Read the model definition and answer for the solid it produces. Units are mm, in the model's axes. A direction names the side the tool comes from. Give positions to 0.01 mm unless a question says otherwise; leave off trailing zeros. Write each loop counter-clockwise with the first axis right and the second up, starting at its lowest first coordinate (ties: lowest second). Pieces come first, ordered by that corner, then holes.
```python
from build123d import *

# Parameters (mm, degrees)
F1_DEPTH      = 3.5
F0_W          = 1.25
F0_H          = 11.5
F2_W          = 21
F2_H          = 11.5
F3_DEPTH      = 2
F4_W          = 27
F4_H          = 14.5
F4_W_2        = 21
F4_H_2        = 5.5
F5_DEPTH      = 11.5
F5_DEPTH_BACK = 4
F6_R          = 1.75
F7_DEPTH      = 25
F9_DEPTH      = 4
F10_R         = 3
F11_DEPTH     = 3
F12_SIZE      = 0.9999
F13_R         = 1.75
F14_DEPTH     = 5


# Not quite as in the source:
# - a fillet or chamfer is up to 0.001 mm smaller than in the source, because OpenCascade refuses the exact size


with BuildPart() as f1:
    # F0 (on Top) → F1 (new body)
    with BuildSketch(Plane.XY):
        Polygon((1.25, 0), (0, 0), (-1.25, 0), (-1.25, -11.5), (0, -11.5), (1.25, -11.5), align=None)
    extrude(amount=F1_DEPTH)



with BuildPart() as f1b:
    # F0 (on Top) → F1, piece 2 (new body)
    with BuildSketch(Plane.XY):
        with Locations((-9.875, -5.75)):
            Rectangle(F0_W, F0_H)
    extrude(amount=F1_DEPTH)


with BuildPart() as f1c:
    # F0 (on Top) → F1, piece 3 (new body)
    with BuildSketch(Plane.XY):
        with Locations((9.875, -5.75)):
            Rectangle(F0_W, F0_H)
    extrude(amount=F1_DEPTH)


with BuildPart() as f1_1:
    add(f1.part)

    add(f1b.part)  # F3 merges F1b

    add(f1c.part)  # F3 merges F1c
    # F2 (on Top) → F3 (join)
    with BuildSketch(Plane.XY):
        with Locations((0, -5.75)):
            Rectangle(F2_W, F2_H)
    extrude(amount=-F3_DEPTH)

    # F4 (on Front) → F5 (join, two sides)
    with BuildSketch(Plane.XZ) as f5_sk:
        with Locations((0, 2.25)):
            Rectangle(F4_W, F4_H)
        with Locations((0, 0.75)):
            Rectangle(F4_W_2, F4_H_2, mode=Mode.SUBTRACT)
    extrude(amount=F5_DEPTH)
    extrude(f5_sk.sketch, amount=-F5_DEPTH_BACK)

    # F6 (on face) → F7 (cut)
    with BuildSketch(Plane.XY):
        with Locations((5.25, -7.5)):
            Circle(F6_R)
        with Locations((-5.25, -7.5)):
            Circle(F6_R)
    extrude(amount=F7_DEPTH, mode=Mode.SUBTRACT)

    # F8 (on face) → F9 (cut)
    with BuildSketch(Plane(origin=(0, 0, 3.5), x_dir=(1, 0, 0), z_dir=(0, 0, -1))):
        Polygon((2.25, 5.7679491924), (5.25, 4.0358983849), (8.25, 5.7679491924), (8.25, 9.2320508076), (5.25, 10.9641016151), (2.25, 9.2320508076), align=None)
        Polygon((2.25, 21.0246167397), (2.25, 9.2320508076), (5.25, 10.9641016151), (8.25, 9.2320508076), (8.25, 21.0246167397), align=None)
        Polygon((-2.25, 21.0246167397), (-8.25, 21.0246167397), (-8.25, 9.2320508076), (-8.25, 5.7679491924), (-5.25, 4.0358983849), (-2.25, 5.7679491924), (-2.25, 9.2320508076), align=None)
    extrude(amount=-F9_DEPTH, mode=Mode.SUBTRACT)

    # F10 (on face) → F11 (cut)
    with BuildSketch(Plane.XZ.offset(11.5)):
        with Locations((5.25, 1.75)):
            Circle(F10_R)
        with Locations((-5.25, 1.75)):
            Circle(F10_R)
    extrude(amount=-F11_DEPTH, mode=Mode.SUBTRACT)

    # F12 (size 1 in the source; OpenCascade refuses exactly that, so slightly less here)
    f12_edges = [f1_1.edges().sort_by_distance(p)[0] for p in [
        (-1.25, -11.5, 1.75),
        (-9.25, -11.5, 1.75),
        (-2.031651, -11.5, 0),
        (-8.468349, -11.5, 0),
        (2.031651, -11.5, 0),
        (1.25, -11.5, 1.75),
        (5.25, -11.5, -1.25),
        (8.468349, -11.5, 0),
        (9.25, -11.5, 1.75),
        (-5.25, -11.5, -1.25),
        (-8.25, -11.5, 5.5),
        (-5.25, -11.5, 7.5),
        (-2.25, -11.5, 5.5),
        (2.25, -11.5, 5.5),
        (5.25, -11.5, 7.5),
        (8.25, -11.5, 5.5),
    ]]
    chamfer(f12_edges, length=F12_SIZE)

    # F13 (on face) → F14 (join)
    with BuildSketch(Plane(origin=(0, 0, -5), x_dir=(1, 0, 0), z_dir=(0, 0, -1))):
        with BuildLine():
            Line((13.5, -4), (17.5, -4))
            ThreePointArc((17.5, -4), (25.25, 3.75), (17.5, 11.5))
            Line((17.5, 11.5), (13.5, 11.5))
            Line((13.5, 11.5000000001), (13.5, -4))
        make_face()
        with Locations((17.5, 3.75)):
            Circle(F13_R, mode=Mode.SUBTRACT)
        with BuildLine():
            ThreePointArc((-17.5, 11.5), (-25.25, 3.75), (-17.5, -4))
            Line((-17.5, -4), (-13.5, -4))
            Line((-13.5, -4), (-13.5, 11.5000000001))
            Line((-13.5, 11.5), (-17.5, 11.5))
        make_face()
        with Locations((-17.5, 3.75)):
            Circle(F13_R, mode=Mode.SUBTRACT)
    extrude(amount=-F14_DEPTH)


solid = f1_1.part
```
Item 1: Determine the mould class of faces 5 (the flat face through (0, -4, 9.5)), 6 (the flat face through (-6.771, -4.914, 5.472)), 7 (the flat face through (-3.77, -4.89, 5.47)) for opening direction X: pulls with the +X half, pulls with the -X half, needs draft (parallel to the pull), parting line crosses it, or undercut.
Result set:
face 5: needs draft
face 6: undercut
face 7: undercut
Item 2: Find the intervals of material crossed by line 1 along X through (y, z) = (-7.5, 8); line 2 along X through (y, z) = (-3.75, -4); line 3 along Y through (x, z) = (17.5, -3.8), in increasing order.
Result set:
line 1: x = -13.5 to -7, -3.5 to 3.5, 7 to 13.5
line 2: x = -25.25 to -19.25, -15.75 to 15.75, 19.25 to 25.25
line 3: y = -11.5 to -5.5, -2 to 4
Item 3: Section D-D (y = -9.75) is taken. Write down the section's boundary in (x, z), and give its area (3 significant figures).
Result set:
outline: (-22.41, -5) - (22.41, -5) - (22.41, 0) - (13.5, 0) - (13.5, 9.5) - (-13.5, 9.5) - (-13.5, 0) - (-22.41, 0) - close; hole (-9.25, 0) - (-7.69, 0) arc R3 ccw to (-2.81, 0) - (-1.25, 0) - (-1.25, 3.5) - (-2.25, 3.5) - (-2.25, 7.5) - (-8.25, 7.5) - (-8.25, 3.5) - (-9.25, 3.5) - close; hole (1.25, 0) - (2.81, 0) arc R3 ccw to (7.69, 0) - (9.25, 0) - (9.25, 3.5) - (8.25, 3.5) - (8.25, 7.5) - (2.25, 7.5) - (2.25, 3.5) - (1.25, 3.5) - close
area: 368 mm2
Item 4: Section B-B (y = 3) is taken. Write down the section's boundary in (x, z).
Result set:
outline: (-21.31, -5) - (21.31, -5) - (21.31, 0) - (13.5, 0) - (13.5, 9.5) - (-13.5, 9.5) - (-13.5, 0) - (-21.31, 0) - close; hole (-10.5, -2) - (10.5, -2) - (10.5, 3.5) - (-10.5, 3.5) - close
Item 5: Which of the six approach directions +Z, -Z, +X, -X, +Y, -Y give full straight-line access (tool end or side, diameter ignored) to faces 1 (the flat face through (10.5, 2, 1)), 2 (the flat face through (0, -11.5, 1)), 3 (the flat face through (3.729, -4.914, 5.472)), 4 (the flat face through (1.25, -5, 2))?
Result set:
face 1: +Y
face 2: +Z, -Z, +X, -X, -Y
face 3: -Y
face 4: +Y, -Y
Item 6: Each of these flat-tipped pins is pushed along its axis until it touches: pin 1 Ø7.5 at (y, z) = (-6, 4.5) entering from -X; pin 2 Ø1.5 at (y, z) = (-1, 4.5) entering from +X; pin 3 Ø3 at (y, z) = (-8, 1) entering from +X. Where does it stop, or does it pass through?
Result set:
pin 1: stops at x = -13.5
pin 2: stops at x = 13.5
pin 3: stops at x = 24.59
Item 7: Section A-A (z = 0.75) is taken. Write down the section's boundary in (x, y).
Result set:
outline: (-13.5, -11.5) - (-10.25, -11.5) - (-9.25, -10.5) - (-9.25, 0) - (-10.5, 0) - (-10.5, 4) - (-13.5, 4) - close; (-1.25, -10.5) - (-0.25, -11.5) - (0.25, -11.5) - (1.25, -10.5) - (1.25, 0) - (-1.25, 0) - close; (9.25, -10.5) - (10.25, -11.5) - (13.5, -11.5) - (13.5, 4) - (10.5, 4) - (10.5, 0) - (9.25, 0) - close
Item 8: Section C-C (z = -3.25) is taken. Write down the section's boundary in (x, y), and give its area (3 significant figures).
Result set:
outline: (-17.5, -11.5) - (17.5, -11.5) arc R7.75 ccw to (17.5, 4) - (-17.5, 4) arc R7.75 ccw to start; hole circle Ø3.5 at (-17.5, -3.75); hole circle Ø3.5 at (17.5, -3.75)
area: 712 mm2
